from build123d import *

# Parameters (mm, degrees)
PAD_DEPTH    = 5
SKETCH002_R  = 9.228742
PAD001_DEPTH = 20
POCKET_DEPTH = 15


with BuildPart() as part:
    # Sketch001 → Pad (new body)
    with BuildSketch(Plane.XY):
        Polygon((0, 10), (80, 10), (80, 50), (100, 50), (100, -50), (80, -50), (80, -10), (0, -10), (-80, -10), (-80, -50), (-100, -50), (-100, 50), (-80, 50), (-80, 10), align=None)
    extrude(amount=PAD_DEPTH)

    # Sketch002 → Pad001 (new body)
    with BuildSketch(Plane.XY.offset(5)):
        with Locations((90, 0)):
            Circle(SKETCH002_R)
        with Locations((-90, 0)):
            Circle(SKETCH002_R)
    extrude(amount=PAD001_DEPTH)

    # Sketch003 → Pocket (cut)
    with BuildSketch(Plane.XY.offset(25)):
        Polygon((-87.480573, 3.871152), (-92.092803, 4.117464), (-94.61223, 0.246312), (-92.519427, -3.871152), (-87.907197, -4.117464), (-85.38777, -0.246312), align=None)
    pocket = extrude(amount=-POCKET_DEPTH, mode=Mode.SUBTRACT)

    # Mirrored: Pocket across Sketch003 V_Axis
    add(pocket.mirror(Plane(origin=(0, 0, 25), x_dir=(0, 0, 1), z_dir=(1, 0, 0))), mode=Mode.SUBTRACT)


solid = part.part
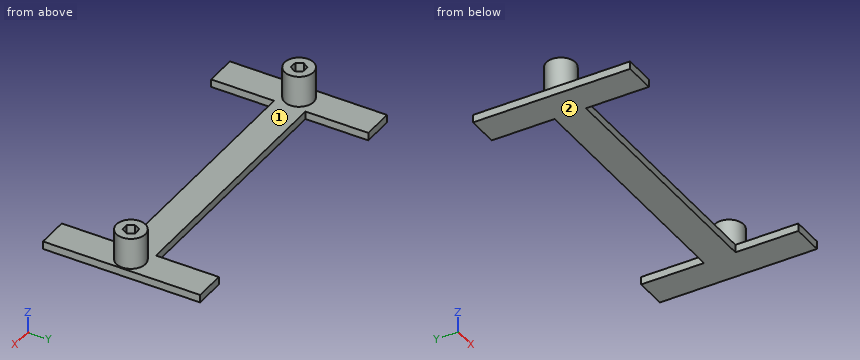
Could you check a few things on this model? Use its own coordinates, in mm. Face numbers are marked on the shaded views. Coordinates: 2 decimals unless noted, no trailing zeros. Order: outer loops, then holes, each group sorted by start corner. A loop starts at its lowest first (then second) coordinate and runs counter-clockwise, first axis right, second up. Notation, with made-up numbers: (31, 77.5) - (73, 77.5) arc R26 ccw to (73, 114.5) - close; hole circle Ø4 at (8.25, 39). An arc over 180 degrees is marked (long way). Answer in a Markdown table with one row per item. Add a question column.
(1) I need wall thicknesses on L1, parallel to X at y = -14, z = 3.75; L2, parallel to X at y = -8, z = 12.25; L3, parallel to Y at x = -5.5, z = 1.5. Which ranges of each line are inside material? Lowest first, please.
(2) If we section it at D-D, the plane x = -90: Please give me the cut outline in (y, z).
(3) If we section it at B-B, the plane y = -29: Please give me the cut outline in (x, z).
(4) Will these pins go through, and if not, where does the flat tip stop? pin 1 (5 mm diameter, centred on x = 21.5, z = 2.5, fed in from -Y); pin 2 (5 mm diameter, centred on y = -26.5, z = 8.5, fed in from +X); pin 3 (4 mm diameter, centred on x = -15, z = 2.5, fed in from +Y); pin 4 (1 mm diameter, centred on y = -6.5, z = 7.5, fed in from +X).
(5) If we section it at C-C, the plane z = 7: Please give me the cut outline in (x, y).
(6) If we mould it in two halves opening along X, with no side actions, what happens to the marked faces 1 and 2? For each: released by +X, released by -X, zero draft, split by the parting line, or undercut.
(7) If we section it at A-A, the plane z = 18: Please give me the cut outline in (x, y), then the cut area to 3 significant figures.
Results are:
| question | item | result |
|---|---|---|
| 1 | L1 | x = -100 to -80, 80 to 100 |
| 1 | L2 | x = -94.6 to -85.4, 85.4 to 94.6 |
| 1 | L3 | y = -10 to 10 |
| 2 | outline | (-50, 0) - (50, 0) - (50, 5) - (9.23, 5) - (9.23, 25) - (4.01, 25) - (4.01, 10) - (-4.01, 10) - (-4.01, 25) - (-9.23, 25) - (-9.23, 5) - (-50, 5) - close |
| 3 | outline | (-100, 0) - (-80, 0) - (-80, 5) - (-100, 5) - close; (80, 0) - (100, 0) - (100, 5) - (80, 5) - close |
| 4 | pin 1 | stops at y = -10 |
| 4 | pin 2 | passes through |
| 4 | pin 3 | stops at y = 10 |
| 4 | pin 4 | stops at x = 97.01 |
| 5 | outline | circle Ø18.46 at (-90, 0); circle Ø18.46 at (90, 0) |
| 6 | face 1 | undercut |
| 6 | face 2 | zero draft |
| 7 | outline | circle Ø18.46 at (-90, 0); circle Ø18.46 at (90, 0); hole (-94.61, 0.25) - (-92.52, -3.87) - (-87.91, -4.12) - (-85.39, -0.25) - (-87.48, 3.87) - (-92.09, 4.12) - close; hole (85.39, -0.25) - (87.91, -4.12) - (92.52, -3.87) - (94.61, 0.25) - (92.09, 4.12) - (87.48, 3.87) - close |
| 7 | area | 424 mm2 |
